Autodesk Inventor part; units mm, degrees
ref_plane "YZ Plane" through (0, 0, 0) normal (1, 0, 0) x (0, 1, 0)
ref_plane "XZ Plane" through (0, 0, 0) normal (0, 1, 0) x (-1, 0, 0)
ref_plane "XY Plane" through (0, 0, 0) normal (0, 0, 1) x (1, 0, 0)
sketch "Boceto1" plane through (0, 0, 0) normal (0, 0, 1) x (1, 0, 0)
  circle A0 centre (0, 0) radius 13.5
  circle A1 centre (0, 0) radius 17.5
  line L0 (17.5, 1.27) -> (17.5, 24.003)
  line L1 (13.5, 1.27) -> (13.5, 20.828)
  line L2 (10.325, 24.003) -> (0, 24.003)
  line L3 (17.5, 24.003) -> (17.5, 24.828)
  line L4 (14.325, 28.003) -> (0, 28.003)
  line L5 (0, 28.003) -> (0, 0)
  arc A2 (17.5, 24.828) -> (14.325, 28.003) centre (14.325, 24.828) ccw
  arc A3 (13.5, 20.828) -> (10.325, 24.003) centre (10.325, 20.828) ccw
  line L6 (16.23, 0) -> (14.77, 0)
  arc A4 (16.23, 0) -> (17.5, 1.27) centre (16.23, 1.27) ccw
  arc A5 (13.5, 1.27) -> (14.77, 0) centre (14.77, 1.27) ccw
  point P0 (17.5, 0)
  point P1 (13.5, 0)
  point P2 (17.5, 28.003)
  dimension "d0" = 27
  dimension "d1" = 35
  dimension "d2" = 24.003
  dimension "d3" = 4
  dimension "d4" = 3.175
  dimension "d5" = 1.27
revolve "Revolución1" add sketch "Boceto1" angle 360 about axis through (0, 28.003, 0) along (0, -1, 0) picked at (14.1771, 6.8232) contours L1 A3 L2 L5 L4 A2 L3 L0 A4 A1 | A1 A4 L6 A5 L1
properties part number "tapap"
Verification items for the finished model (mm, model axes). Give positions to 0.01 mm unless a question says otherwise; leave off trailing zeros. Loops run counter-clockwise (first coordinate to the right, second up) from the corner with the lowest first, then second, coordinate; pieces in that order, holes last. Notation, with made-up numbers: (84.5, 86) - (132.5, 86) arc R19 ccw to (132.5, 92) - close; hole circle Ø1 at (-16.5, -3.5). An arc over 180 degrees is marked (long way). Write item = value, one per line. Start each with the question number.
Q1. Mould release check, pull along X, two halves, no side actions. Record for faces 1 (the face through (0, 28.003, 0)), 2 (the face through (-13.887, 13.214, 10.648)), 3 (the face through (0, 24.003, 0)), 4 (the face through (-2.93, 11.19, 13.18)): released by +X, released by -X, zero draft, split by the parting line, or undercut.
Q2. Cross-section at A-A, the plane z = 0. Enter the section's corners in (x, y) (3 decimals).
Q3. Thickness scan on line 1 (Z direction, x = 0, y = 15.5); line 2 (Z direction, x = 11, y = 16.5); line 3 (Y direction, x = 6.5, z = -3.5). Record the ranges inside material, lowest first.
Q4. Cross-section at C-C, the plane y = 8.75. Enter the section's corners in (x, z).
Q5. Depth check by flat-ended pin: P1, Ø16.5, axis at x = 3.5, z = -3, coming from the -Y side; P2, Ø8, axis at x = -6, y = 25, coming from the +Z side; P3, Ø6, axis at x = 1, z = 11, coming from the -Y side; P4, Ø2, axis at x = 1, y = 17, coming from the +Z side. Enter the tip coordinate at first touch or a pass-through.
Q6. Cross-section at B-B, the plane x = 0. Enter the section's corners in (y, z) (3 decimals), and give its area (3 significant figures).
Answer key:
q1.face_1 = zero draft
q1.face_2 = split by the parting line
q1.face_3 = undercut
q1.face_4 = undercut
q2.outline = (-17.5, 1.27) arc R1.27 ccw to (-16.23, 0) - (-14.77, 0) arc R1.27 ccw to (-13.5, 1.27) - (-13.5, 20.828) arc R3.175 cw to (-10.325, 24.003) - (10.325, 24.003) arc R3.175 cw to (13.5, 20.828) - (13.5, 1.27) arc R1.27 ccw to (14.77, 0) - (16.23, 0) arc R1.27 ccw to (17.5, 1.27) - (17.5, 24.828) arc R3.175 ccw to (14.325, 28.003) - (-14.325, 28.003) arc R3.175 ccw to (-17.5, 24.828) - close
q3.line_1 = -17.5 to -13.5, 13.5 to 17.5
q3.line_2 = -13.61 to -7.83, 7.83 to 13.61
q3.line_3 = 24 to 28
q4.outline = circle Ø35 at (0, 0); hole circle Ø27 at (0, 0)
q5.P1 = 22.74
q5.P2 = 17.38
q5.P3 = 0.23
q5.P4 = 17.5
q6.outline = (0, -16.23) arc R1.27 ccw to (1.27, -17.5) - (24.828, -17.5) arc R3.175 ccw to (28.003, -14.325) - (28.003, 14.325) arc R3.175 ccw to (24.828, 17.5) - (1.27, 17.5) arc R1.27 ccw to (0, 16.23) - (0, 14.77) arc R1.27 ccw to (1.27, 13.5) - (20.828, 13.5) arc R3.175 cw to (24.003, 10.325) - (24.003, -10.325) arc R3.175 cw to (20.828, -13.5) - (1.27, -13.5) arc R1.27 ccw to (0, -14.77) - close
q6.area = 331 mm^2
